from build123d import *

# Parameters (mm, degrees)
F0_W      = 63.5
F0_H      = 50.8
F1_DEPTH  = 38.1
F2_SIZE   = 5.08
F3_R      = 3.175
F4_DEPTH  = 12.7
F5_W      = 30.805484
F5_H      = 29.21
F6_DEPTH  = 1.27
F7_W      = 12.203076
F7_H      = 12.192
F8_DEPTH  = 1.27
F9_W      = 2.545274
F9_H      = 0.933269
F9_W_2    = 2.545275
F10_DEPTH = 0.762


with BuildPart() as f1:
    # F0 (on Top) → F1 (new body)
    with BuildSketch(Plane.XY):
        with Locations((-2.185041, -0.428895)):
            Rectangle(F0_W, F0_H)
    extrude(amount=F1_DEPTH)

    # F2
    f2_edges = [f1.edges().sort_by_distance(p)[0] for p in [
        (-33.935041, -0.428895, 38.1),
        (-2.185041, -25.828895, 38.1),
        (29.564959, -0.428895, 38.1),
        (-2.185041, 24.971105, 38.1),
    ]]
    chamfer(f2_edges, length=F2_SIZE)

    # F3 (on face) → F4 (cut)
    with BuildSketch(Plane(origin=(-33.935041, 0, 0), x_dir=(0, -1, 0), z_dir=(-1, 0, 0))):
        with Locations((0, 16.51)):
            Circle(F3_R)
    extrude(amount=-F4_DEPTH, mode=Mode.SUBTRACT)

    # F5 (on face) → F6 (cut)
    with BuildSketch(Plane.XZ.offset(25.828895)):
        with Locations((-16.627299, 16.51)):
            Rectangle(F5_W, F5_H)
    extrude(amount=-F6_DEPTH, mode=Mode.SUBTRACT)

    # F7 (on face) → F8 (join)
    with BuildSketch(Plane.XZ.offset(24.558895)):
        with Locations((-24.658503, 23.749)):
            Rectangle(F7_W, F7_H)
        with Locations((-8.606803, 23.749)):
            Rectangle(F7_W, F7_H)
        with Locations((-24.606782, 9.18722)):
            Rectangle(F7_W, F7_H)
        with Locations((-8.555082, 9.18722)):
            Rectangle(F7_W, F7_H)
    extrude(amount=F8_DEPTH)

    # F9 (on face) → F10 (join)
    with BuildSketch(Plane.XZ.offset(25.828895)):
        with Locations((-28.48023, 28.082971)):
            Rectangle(F9_W, F9_H)
        with Locations((-24.67023, 28.082971)):
            Rectangle(F9_W, F9_H)
        with Locations((-20.86023, 28.082971)):
            Rectangle(F9_W, F9_H)
        with Locations((-28.448142, 24.052954)):
            Rectangle(F9_W_2, F9_H)
        with Locations((-24.638143, 24.052954)):
            Rectangle(F9_W_2, F9_H)
        with Locations((-20.828142, 24.052954)):
            Rectangle(F9_W_2, F9_H)
        with Locations((-20.796056, 20.022937)):
            Rectangle(F9_W_2, F9_H)
        with Locations((-24.606055, 20.022937)):
            Rectangle(F9_W_2, F9_H)
        with Locations((-28.416055, 20.022937)):
            Rectangle(F9_W_2, F9_H)
        with Locations((-28.702667, 13.362789)):
            Rectangle(F9_W_2, F9_H)
        with Locations((-24.892668, 13.362789)):
            Rectangle(F9_W_2, F9_H)
        with Locations((-21.082667, 13.362789)):
            Rectangle(F9_W_2, F9_H)
        with Locations((-21.05058, 9.332771)):
            Rectangle(F9_W, F9_H)
        with Locations((-24.86058, 9.332771)):
            Rectangle(F9_W, F9_H)
        with Locations((-28.67058, 9.332771)):
            Rectangle(F9_W, F9_H)
        with Locations((-28.638492, 5.302754)):
            Rectangle(F9_W_2, F9_H)
        with Locations((-24.828492, 5.302754)):
            Rectangle(F9_W_2, F9_H)
        with Locations((-21.018493, 5.302754)):
            Rectangle(F9_W_2, F9_H)
        with Locations((-12.518417, 9.247929)):
            Rectangle(F9_W_2, F9_H)
        with Locations((-12.550504, 13.277945)):
            Rectangle(F9_W_2, F9_H)
        with Locations((-8.740505, 13.277945)):
            Rectangle(F9_W_2, F9_H)
        with Locations((-8.708417, 9.247929)):
            Rectangle(F9_W_2, F9_H)
        with Locations((-4.898417, 9.247929)):
            Rectangle(F9_W_2, F9_H)
        with Locations((-4.930504, 13.277945)):
            Rectangle(F9_W_2, F9_H)
        with Locations((-4.86633, 5.217911)):
            Rectangle(F9_W, F9_H)
        with Locations((-8.67633, 5.217911)):
            Rectangle(F9_W, F9_H)
        with Locations((-12.48633, 5.217911)):
            Rectangle(F9_W, F9_H)
        with Locations((-12.328067, 27.998128)):
            Rectangle(F9_W_2, F9_H)
        with Locations((-8.518067, 27.998128)):
            Rectangle(F9_W_2, F9_H)
        with Locations((-4.708067, 27.998128)):
            Rectangle(F9_W_2, F9_H)
        with Locations((-4.67598, 23.968111)):
            Rectangle(F9_W, F9_H)
        with Locations((-8.48598, 23.968111)):
            Rectangle(F9_W, F9_H)
        with Locations((-12.29598, 23.968111)):
            Rectangle(F9_W, F9_H)
        with Locations((-12.263892, 19.938094)):
            Rectangle(F9_W_2, F9_H)
        with Locations((-8.453893, 19.938094)):
            Rectangle(F9_W_2, F9_H)
        with Locations((-4.643892, 19.938094)):
            Rectangle(F9_W_2, F9_H)
    extrude(amount=F10_DEPTH)


solid = f1.part
Can you work these out from the model? Positions are in its coordinate system, mm. A direction names the side the tool comes from. Round coordinates to 2 decimals unless told otherwise and drop trailing zeros. Write each loop counter-clockwise with the first axis right and the second up, starting at its lowest first coordinate (ties: lowest second). Pieces come first, ordered by that corner, then holes. Notation, with made-up numbers: (42, 42) - (54, 42) arc R10 ccw to (54, 59) - close; hole circle Ø3 at (-2, 12.25). An arc over 180 degrees is marked (long way). Write each question's results on one line, items separated by ' | '. Start each with the question number.
1) Suppose I cut it at A-A (z = 16.51). List the corners of the cut face in (x, y) for me (3 decimals), and give its area (3 significant figures).
2) Please list where these lines run through material, in increasing order: line 1 (Z direction, x = -24, y = 0) (3 decimals); line 2 (Y direction, x = -24, z = 27); line 3 (Z direction, x = -29, y = 0) (3 decimals).
3) For pin 1 Ø1 at (x, z) = (22.5, 8) entering from -Y; pin 2 Ø0.8 at (y, z) = (-26.5, 13.5) entering from +X; pin 3 Ø0.6 at (y, z) = (-26.5, 9.5) entering from +X; pin 4 Ø0.6 at (x, y) = (-20.5, -26) entering from -Z, each with a flat end and sliding along its axis, tell me the tip position at first contact or that it passes through.
4) Suppose I cut it at B-B (y = 0). List the corners of the cut face in (x, z) for me (3 decimals).
5) We'd pull the mould along Z, two halves only. Please class faces 1 (the flat face through (-31.359, -0.784, 35.596)), 2 (the flat face through (-25, -25.829, 11)), 3 (the flat face through (-18, -24.559, 17)), 4 (the flat face through (29.565, -1, 16)): released by +Z, released by -Z, zero draft, split by the parting line, or undercut.
6) Suppose I cut it at D-D (z = 8). List the corners of the cut face in (x, y) for me.
7) Suppose I cut it at C-C (x = 6.5). List the corners of the cut face in (y, z) for me.
8) Which directions (+Z, -Z, +X, -X, +Y, -Y) give clear straight access to the entire face, cutting with the end or side of a thin tool? Please do faces 5 (the flat face through (-3, 24.971, 16)), 6 (the cylindrical face through (-27.67, 0.41, 19.66)).
Here are the results:
1) outline: (-33.935, -25.829) - (-32.03, -25.829) - (-32.03, -24.559) - (-1.225, -24.559) - (-1.225, -25.829) - (29.565, -25.829) - (29.565, 24.971) - (-33.935, 24.971) - (-33.935, 3.175) - (-21.235, 3.175) - (-21.235, -3.175) - (-33.935, -3.175) - close | area: 3,110 mm2
2) line 1: z = 0 to 13.335, 19.685 to 38.1 | line 2: y = -25.83 to 24.97 | line 3: z = 0 to 13.335, 19.685 to 37.955
3) pin 1: stops at y = -25.83 | pin 2: stops at x = -3.66 | pin 3: stops at x = -3.63 | pin 4: stops at z = 0
4) outline: (-33.935, 0) - (29.565, 0) - (29.565, 33.02) - (24.485, 38.1) - (-28.855, 38.1) - (-33.935, 33.02) - (-33.935, 19.685) - (-21.235, 19.685) - (-21.235, 13.335) - (-33.935, 13.335) - close
5) face 1: released by +Z | face 2: undercut | face 3: undercut | face 4: zero draft
6) outline: (-33.94, -25.83) - (-32.03, -25.83) - (-32.03, -24.56) - (-30.71, -24.56) - (-30.71, -25.83) - (-18.51, -25.83) - (-18.51, -24.56) - (-14.66, -24.56) - (-14.66, -25.83) - (-2.45, -25.83) - (-2.45, -24.56) - (-1.22, -24.56) - (-1.22, -25.83) - (29.56, -25.83) - (29.56, 24.97) - (-33.94, 24.97) - close
7) outline: (-25.83, 0) - (24.97, 0) - (24.97, 33.02) - (19.89, 38.1) - (-20.75, 38.1) - (-25.83, 33.02) - close
8) face 5: +Z, -Z, +X, -X, +Y | face 6: -X
